Geometry check sheet. Reference: the model listing, model coordinates, mm. A direction names the side the tool comes from. Coordinates: 2 decimals unless noted, no trailing zeros. Order: outer loops, then holes, each group sorted by start corner. A loop starts at its lowest first (then second) coordinate and runs counter-clockwise, first axis right, second up. Notation, with made-up numbers: (75.5, -19) - (97.5, -19) arc R17 cw to (97.5, -15) - close; hole circle Ø2 at (63, -26). An arc over 180 degrees is marked (long way). One line per item, written item: value. Start each with the question number.
```python
from build123d import *

# Parameters (mm, degrees)
BODY_S_W      = 10.4
BODY_S_H      = 6.3
BODY_DEPTH    = 1.8
EDGE_FILLET_R = 0.3
BASE_S_W      = 11.8
BASE_S_H      = 7.7
BASE_DEPTH    = 3.2
PEG_S_W       = 4
PEG_S_H       = 3
PEG_DEPTH     = 2.5


with BuildPart() as part:
    # body-s → body (new body)
    with BuildSketch(Plane(origin=(0, 0, 0), x_dir=(1, 0, 0), z_dir=(0, 1, 0))):
        Rectangle(BODY_S_W, BODY_S_H)
    extrude(amount=BODY_DEPTH)

    # edge-fillet
    edge_fillet_edges = [part.edges().sort_by_distance(p)[0] for p in [
        (5.2, 0.9, 3.15),
        (-5.2, 0.9, 3.15),
        (-5.2, 0.9, -3.15),
        (5.2, 0.9, -3.15),
    ]]
    fillet(edge_fillet_edges, radius=EDGE_FILLET_R)

    # base-s → base (add)
    with BuildSketch(Plane.XZ):
        Rectangle(BASE_S_W, BASE_S_H)
    extrude(amount=BASE_DEPTH)

    # peg-s → peg (add)
    with BuildSketch(Plane.XZ.offset(3.2)):
        Rectangle(PEG_S_W, PEG_S_H)
    extrude(amount=PEG_DEPTH)


solid = part.part
```
Q1. Set-up check for faces 1 (the flat face through (-2, -4, 0)), 2 (the flat face through (0, 1, -3.15)), 3 (the flat face through (0, 1, 3.15)), 4 (the flat face through (-5.2, 1, 0)): record each of +Z, -Z, +X, -X, +Y, -Y from which the full face is reachable in a straight line by a thin tool's end or side.
Q2. Material ranges on probe 1 along Y at (x, z) = (-1.75, -2); probe 2 along X at (y, z) = (-4, -1); probe 3 along Z at (x, y) = (2, 1.5), recorded low to high.
Q3. Cross-section at D-D, the plane x = 3.75. Enter the section's corners in (y, z), and give its area (3 significant figures).
Q4. Cross-section at A-A, the plane x = -1.5. Enter the section's corners in (y, z), and give its area (3 significant figures).
Q5. Cross-section at B-B, the plane z = -0.25. Enter the section's corners in (x, y), and give its area (3 significant figures).
Q6. Gauge pin test, flat ends, axial feed: P1, Ø1.2, axis at y = -4, z = 0, coming from the -X side; P2, Ø0.9, axis at x = -0.5, y = 0.5, coming from the +Z side; P3, Ø2, axis at x = -1, y = -5, coming from the -Z side. Record the tip position at first contact, or that the pin passes through.
Q7. Cross-section at C-C, the plane y = 0.25. Enter the section's corners in (x, z), and give its area (3 significant figures).
Check result:
1. face 1: +Z, -Z, -X, -Y
1. face 2: -Z, +X, -X, +Y
1. face 3: +Z, +X, -X, +Y
1. face 4: +Z, -Z, -X, +Y
2. probe 1: y = -3.2 to 1.8
2. probe 2: x = -2 to 2
2. probe 3: z = -3.15 to 3.15
3. outline: (-3.2, -3.85) - (0, -3.85) - (0, -3.15) - (1.8, -3.15) - (1.8, 3.15) - (0, 3.15) - (0, 3.85) - (-3.2, 3.85) - close
3. area: 36.0 mm2
4. outline: (-5.7, -1.5) - (-3.2, -1.5) - (-3.2, -3.85) - (0, -3.85) - (0, -3.15) - (1.8, -3.15) - (1.8, 3.15) - (0, 3.15) - (0, 3.85) - (-3.2, 3.85) - (-3.2, 1.5) - (-5.7, 1.5) - close
4. area: 43.5 mm2
5. outline: (-5.9, -3.2) - (-2, -3.2) - (-2, -5.7) - (2, -5.7) - (2, -3.2) - (5.9, -3.2) - (5.9, 0) - (5.2, 0) - (5.2, 1.8) - (-5.2, 1.8) - (-5.2, 0) - (-5.9, 0) - close
5. area: 66.5 mm2
6. P1: stops at x = -2
6. P2: stops at z = 3.15
6. P3: stops at z = -1.5
7. outline: (-5.2, -2.85) arc R0.3 ccw to (-4.9, -3.15) - (4.9, -3.15) arc R0.3 ccw to (5.2, -2.85) - (5.2, 2.85) arc R0.3 ccw to (4.9, 3.15) - (-4.9, 3.15) arc R0.3 ccw to (-5.2, 2.85) - close
7. area: 65.4 mm2
